Check sheet for the modelled part. Datum: model origin and axes. Units: mm. A direction names the side the tool comes from. Round coordinates to 2 decimals unless told otherwise and drop trailing zeros. Write each loop counter-clockwise with the first axis right and the second up, starting at its lowest first coordinate (ties: lowest second). Pieces come first, ordered by that corner, then holes. Notation, with made-up numbers: (15.25, -1.5) -> (42.25, -1.5) arc R30 cw to (42.25, 24.5) -> close; hole circle Ø4 at (83, 41.5). An arc over 180 degrees is marked (long way). One line per item, written item: value.
from build123d import *

# Parameters (mm, degrees)
BASEPLATE_OUTLINE_R = 2.1
BASEPLATE_DEPTH     = 2.8
CUT_EXTRUDE1_REACH  = 115.438
SKETCH3_W           = 15.4
SKETCH3_H           = 19.2
SKETCH3_W_2         = 15.6
SKETCH3_W_3         = 16.2
SKETCH3_H_2         = 24


# Read off the part's stored shape, not the designer's step: BasePlate
with BuildPart() as part:
    # BasePlate outline → BasePlate (new body)
    with BuildSketch(Plane(origin=(0, 0, 0), x_dir=(1, 0, 0), z_dir=(0, 1, 0))):
        with BuildLine():
            Line((43.502626614, -5.852332608), (48.792614178, -5.852332608))
            ThreePointArc((48.792614178, -5.852332608), (49.082078508, -5.760021707), (49.264659986, -5.517174213))
            Line((49.264659986, -5.517174213), (50.078201202, -3.187491002))
            ThreePointArc((50.078201202, -3.187491002), (50.26078268, -2.944643509), (50.55024701, -2.852332608))
            Line((50.55024701, -2.852332608), (58.116695703, -2.852332608))
            ThreePointArc((58.116695703, -2.852332608), (58.484685739, -3.013831008), (58.614956567, -3.393999275))
            ThreePointArc((58.614956567, -3.393999275), (64.799237397, -7.61016844), (65.229166667, -0.137781095))
            ThreePointArc((65.229166667, -0.137781095), (65.061014427, 0.043158816), (65, 0.282515593))
            Line((65, 0.282515593), (65, 83.012819192))
            ThreePointArc((65, 83.012819192), (65.061014427, 83.252175969), (65.229166667, 83.433115879))
            ThreePointArc((65.229166667, 83.433115879), (65.940559159, 90.088226551), (59.285448487, 89.376834059))
            ThreePointArc((59.285448487, 89.376834059), (59.104508577, 89.208681819), (58.8651518, 89.147667392))
            Line((58.8651518, 89.147667392), (6.1348482, 89.147667392))
            ThreePointArc((6.1348482, 89.147667392), (5.895491423, 89.208681819), (5.714551513, 89.376834059))
            ThreePointArc((5.714551513, 89.376834059), (-0.940559159, 90.088226551), (-0.229166667, 83.433115879))
            ThreePointArc((-0.229166667, 83.433115879), (-0.061014427, 83.252175969), (0, 83.012819192))
            Line((0, 83.012819192), (0, 0.282515593))
            ThreePointArc((0, 0.282515593), (-0.061014427, 0.043158816), (-0.229166667, -0.137781095))
            ThreePointArc((-0.229166667, -0.137781095), (0.200762603, -7.61016844), (6.385043433, -3.393999275))
            ThreePointArc((6.385043433, -3.393999275), (6.515314261, -3.013831008), (6.883304297, -2.852332608))
            Line((6.883304297, -2.852332608), (14.44975299, -2.852332608))
            ThreePointArc((14.44975299, -2.852332608), (14.73921732, -2.944643509), (14.921798798, -3.187491002))
            Line((14.921798798, -3.187491002), (15.735340014, -5.517174213))
            ThreePointArc((15.735340014, -5.517174213), (15.917921492, -5.760021707), (16.207385822, -5.852332608))
            Line((16.207385822, -5.852332608), (21.497373386, -5.852332608))
            ThreePointArc((21.497373386, -5.852332608), (21.786837716, -5.760021707), (21.969419194, -5.517174213))
            Line((21.969419194, -5.517174213), (22.78296041, -3.187491002))
            ThreePointArc((22.78296041, -3.187491002), (22.965541888, -2.944643509), (23.255006218, -2.852332608))
            Line((23.255006218, -2.852332608), (41.744993782, -2.852332608))
            ThreePointArc((41.744993782, -2.852332608), (42.034458112, -2.944643509), (42.21703959, -3.187491002))
            Line((42.21703959, -3.187491002), (43.030580806, -5.517174213))
            ThreePointArc((43.030580806, -5.517174213), (43.213162284, -5.760021707), (43.502626614, -5.852332608))
        make_face()
        with Locations((2.1, -3.752332608)):
            Circle(BASEPLATE_OUTLINE_R, mode=Mode.SUBTRACT)
        with Locations((62.9, -3.752332608)):
            Circle(BASEPLATE_OUTLINE_R, mode=Mode.SUBTRACT)
        with Locations((2.1, 87.047667392)):
            Circle(BASEPLATE_OUTLINE_R, mode=Mode.SUBTRACT)
        with Locations((62.9, 87.047667392)):
            Circle(BASEPLATE_OUTLINE_R, mode=Mode.SUBTRACT)
    extrude(amount=BASEPLATE_DEPTH)

    # Sketch3 → Cut-Extrude1 (cut, up to next)
    with BuildSketch(Plane(origin=(0, 2.8, 0), x_dir=(1, 0, 0), z_dir=(0, 1, 0)), mode=Mode.PRIVATE) as cut_extrude1_sk1:
        Polygon((4.8, 1.147667392), (59, 1.147667392), (59, 42.447667392), (61, 42.447667392), (61, 46.147667392), (59, 46.147667392), (59, 57.147667392), (35.4, 57.147667392), (35.4, 61.647667392), (33.1, 61.647667392), (33.1, 66.147667392), (19.8, 66.147667392), (19.8, 61.647667392), (4.8, 61.647667392), align=None)
    cut_extrude1_tool1 = extrude(cut_extrude1_sk1.sketch, amount=-CUT_EXTRUDE1_REACH, mode=Mode.PRIVATE) & part.part
    # Sketch3 → Cut-Extrude1 (cut, up to next)
    with BuildSketch(Plane(origin=(0, 2.8, 0), x_dir=(1, 0, 0), z_dir=(0, 1, 0)), mode=Mode.PRIVATE) as cut_extrude1_sk2:
        with Locations((14, 79.547667392)):
            Rectangle(SKETCH3_W, SKETCH3_H)
    cut_extrude1_tool2 = extrude(cut_extrude1_sk2.sketch, amount=-CUT_EXTRUDE1_REACH, mode=Mode.PRIVATE) & part.part
    # Sketch3 → Cut-Extrude1 (cut, up to next)
    with BuildSketch(Plane(origin=(0, 2.8, 0), x_dir=(1, 0, 0), z_dir=(0, 1, 0)), mode=Mode.PRIVATE) as cut_extrude1_sk3:
        with Locations((32, 79.547667392)):
            Rectangle(SKETCH3_W_2, SKETCH3_H)
    cut_extrude1_tool3 = extrude(cut_extrude1_sk3.sketch, amount=-CUT_EXTRUDE1_REACH, mode=Mode.PRIVATE) & part.part
    # Sketch3 → Cut-Extrude1 (cut, up to next)
    with BuildSketch(Plane(origin=(0, 2.8, 0), x_dir=(1, 0, 0), z_dir=(0, 1, 0)), mode=Mode.PRIVATE) as cut_extrude1_sk4:
        with Locations((51, 77.147667392)):
            Rectangle(SKETCH3_W_3, SKETCH3_H_2)
    cut_extrude1_tool4 = extrude(cut_extrude1_sk4.sketch, amount=-CUT_EXTRUDE1_REACH, mode=Mode.PRIVATE) & part.part
    add(cut_extrude1_tool1.solids().sort_by_distance((31.36203, 2.8, -31.109713))[0], mode=Mode.SUBTRACT)
    add(cut_extrude1_tool2.solids().sort_by_distance((14, 2.8, -79.547667))[0], mode=Mode.SUBTRACT)
    add(cut_extrude1_tool3.solids().sort_by_distance((32, 2.8, -79.547667))[0], mode=Mode.SUBTRACT)
    add(cut_extrude1_tool4.solids().sort_by_distance((51, 2.8, -77.147667))[0], mode=Mode.SUBTRACT)


solid = part.part
Item 1: Sectioned sample at A-A (x = 56.5). Enter the section's corners in (y, z).
Result set:
outline: (0, -65.15) -> (2.8, -65.15) -> (2.8, -57.15) -> (0, -57.15) -> close; (0, -1.15) -> (2.8, -1.15) -> (2.8, 2.85) -> (0, 2.85) -> close
Item 2: Tool access check on faces 1 (the flat face through (6.3, 1, -79)), 2 (the flat face through (43, 0, -60)), 3 (the flat face through (0, 1, -42)), 4 (the flat face through (35.4, 1, -59)), 5 (the flat face through (15.323, 1.38, 4.336)). Record the directions out of +Z, -Z, +X, -X, +Y, -Y that give a thin tool (end or side, any length) a straight path to the whole face; none if there is none.
Result set:
face 1: -Z, +Y, -Y
face 2: +Z, -Z, +X, -X, -Y
face 3: -X, +Y, -Y
face 4: +Y, -Y
face 5: +Z, +Y, -Y
Item 3: Sectioned sample at C-C (x = 2.1). Enter the section's corners in (y, z).
Result set:
outline: (0, -91.35) -> (2.8, -91.35) -> (2.8, -89.15) -> (0, -89.15) -> close; (0, -84.95) -> (2.8, -84.95) -> (2.8, 1.65) -> (0, 1.65) -> close; (0, 5.85) -> (2.8, 5.85) -> (2.8, 8.05) -> (0, 8.05) -> close
Item 4: Release check for a two-part mould opening along Z. For faces 6 (the cylindrical face through (64.903, 1.38, 3.122)), 7 (the flat face through (41, 1, -89.148)), 8 (the flat face through (46, 1, 5.852)) record: pulls with the +Z half, pulls with the -Z half, needs draft (parallel to the pull), parting line crosses it, or undercut.
Result set:
face 6: undercut
face 7: pulls with the -Z half
face 8: pulls with the +Z half
Item 5: Sectioned sample at D-D (z = -26.5). Enter the section's corners in (x, y), then the cut area to 3 significant figures.
Result set:
outline: (0, 0) -> (4.8, 0) -> (4.8, 2.8) -> (0, 2.8) -> close; (59, 0) -> (65, 0) -> (65, 2.8) -> (59, 2.8) -> close
area: 30.2 mm^2
Item 6: Material ranges on line 1 along Z through (x, y) = (2.1, 1.35); line 2 along X through (y, z) = (2.7, -75.5), recorded low to high.
Result set:
line 1: -91.35 to -89.15, -84.95 to 1.65, 5.85 to 8.05
line 2: 0 to 6.3, 21.7 to 24.2, 39.8 to 42.9, 59.1 to 65
Item 7: Depth check by flat-ended pin: pin 1 (10 mm diameter, centred on x = 5.5, z = -51, fed in from -Y); pin 2 (0.8 mm diameter, centred on x = 47.5, y = 2, fed in from +Z); pin 3 (1.4 mm diameter, centred on y = 1.5, z = -73.5, fed in from -X); pin 4 (1.4 mm diameter, centred on x = 37, y = 1, fed in from +Z). Enter the tip coordinate at first touch or a pass-through.
Result set:
pin 1: y = 0
pin 2: z = 5.85
pin 3: x = 0
pin 4: z = 2.85
Item 8: Sectioned sample at B-B (z = -82). Enter the section's corners in (x, y).
Result set:
outline: (0, 0) -> (6.3, 0) -> (6.3, 2.8) -> (0, 2.8) -> close; (21.7, 0) -> (24.2, 0) -> (24.2, 2.8) -> (21.7, 2.8) -> close; (39.8, 0) -> (42.9, 0) -> (42.9, 2.8) -> (39.8, 2.8) -> close; (59.1, 0) -> (65, 0) -> (65, 2.8) -> (59.1, 2.8) -> close
